Geometry: final body of the model. Coordinates: model frame, mm. Face numbers are marked on the shaded views. A direction names the side the tool comes from. Coordinates: 2 decimals unless noted, no trailing zeros. Loops run counter-clockwise (first coordinate to the right, second up) from the corner with the lowest first, then second, coordinate; pieces in that order, holes last. Notation, with made-up numbers: (12.5, 23) - (68.5, 23) arc R19 ccw to (68.5, 35) - close; hole circle Ø6 at (29.25, -0.5). An arc over 180 degrees is marked (long way). Put each result on its own line as item: value. Start each with the question number.
1) Reachability of the marked faces 1, 2 and 3 from +Z, -Z, +X, -X, +Y, -Y: full face, straight path, thin tool, end or side. Return the list, or none.
2) Contact query for flat-ended pins moving along their axis: pin 1 Ø3 at (y, z) = (9, -25.5) entering from -X; pin 2 Ø10 at (y, z) = (34.5, -19) entering from -X; pin 3 Ø6 at (y, z) = (32, -29) entering from +X; pin 4 Ø3.5 at (x, z) = (61.5, -20) entering from +Y. Output: stop coordinate, or through.
3) Material intervals for line 1 along X through (y, z) = (1, -20); line 2 along X through (y, z) = (39.75, -20); line 3 along Z through (x, y) = (50, 3), sorted ascending. Write a range as from..to.
4) Section D-D on y = 43.5. Output: boundary loops of the cut face in (x, z).
5) Draft query along Y for the marked faces 4, 5, 6 and 7. Return one class per face: +Y half, -Y half, draft (parallel to the pull), parting line (faces both ways), or undercut.
6) Section B-B on x = 35. Output: boundary loops of the cut face in (y, z).
7) Section C-C on y = 29. Output: boundary loops of the cut face in (x, z), and give its area (3 significant figures).
8) Section A-A on z = -20. Output: boundary loops of the cut face in (x, y), and give its area (3 significant figures).
```python
from build123d import *

# Parameters (mm, degrees)
BOSS_EXTRUDE1_DEPTH = 7
SKETCH4_R           = 1.55
CUT_EXTRUDE1_DEPTH  = 89.684835231
SKETCH5_W           = 70
SKETCH5_H           = 8
BOSS_EXTRUDE2_DEPTH = 40
SKETCH6_W           = 20
SKETCH6_H           = 20
CUT_EXTRUDE2_DEPTH  = 101.124921973
BOSS_EXTRUDE4_DEPTH = 46
SKETCH9_R           = 2.6
CUT_EXTRUDE3_DEPTH  = 101.124921973
SKETCH10_W          = 70
SKETCH10_H          = 7
BOSS_EXTRUDE5_DEPTH = 7


with BuildPart() as part:
    # Sketch1 → Boss-Extrude1 (new body)
    with BuildSketch(Plane(origin=(0, 0, 0), x_dir=(1, 0, 0), z_dir=(0, 1, 0))):
        Polygon((0, 54), (0, 0), (15, 0), (15, 41), (55, 41), (55, 0), (70, 0), (70, 54), align=None)
    extrude(amount=BOSS_EXTRUDE1_DEPTH)

    # Sketch4 → Cut-Extrude1 (cut, through all)
    with BuildSketch(Plane(origin=(0, 7, 0), x_dir=(1, 0, 0), z_dir=(0, 1, 0))):
        with Locations(Location((8.5, 20, 0), (0, 0, 270))):
            Circle(SKETCH4_R)
        with Locations(Location((61.5, 20, 0), (0, 0, 270))):
            Circle(SKETCH4_R)
    extrude(amount=-CUT_EXTRUDE1_DEPTH, mode=Mode.SUBTRACT)

    # Sketch5 → Boss-Extrude2 (add)
    with BuildSketch(Plane(origin=(0, 7, 0), x_dir=(1, 0, 0), z_dir=(0, 1, 0))):
        with Locations((35, 50)):
            Rectangle(SKETCH5_W, SKETCH5_H)
    extrude(amount=BOSS_EXTRUDE2_DEPTH)

    # Sketch6 → Cut-Extrude2 (cut, through all)
    with BuildSketch(Plane(origin=(0, 0, -54), x_dir=(-1, 0, 0), z_dir=(0, 0, -1))):
        with Locations((-35, 27)):
            Rectangle(SKETCH6_W, SKETCH6_H)
    extrude(amount=-CUT_EXTRUDE2_DEPTH, mode=Mode.SUBTRACT)

    # Sketch8 → Boss-Extrude4 (add)
    with BuildSketch(Plane.XY.offset(-46)):
        Polygon((18, 47), (52, 47), (52, 27), (45, 27), (45, 37), (25, 37), (25, 27), (18, 27), align=None)
    extrude(amount=BOSS_EXTRUDE4_DEPTH)

    # Sketch9 → Cut-Extrude3 (cut, through all)
    with BuildSketch(Plane(origin=(0, 47, 0), x_dir=(1, 0, 0), z_dir=(0, 1, 0))):
        with Locations(Location((35, 20, 0), (0, 0, 270))):
            Circle(SKETCH9_R)
    extrude(amount=-CUT_EXTRUDE3_DEPTH, mode=Mode.SUBTRACT)

    # Sketch10 → Boss-Extrude5 (add)
    with BuildSketch(Plane.XY):
        with Locations((35, 3.5)):
            Rectangle(SKETCH10_W, SKETCH10_H)
    extrude(amount=BOSS_EXTRUDE5_DEPTH)


solid = part.part
```
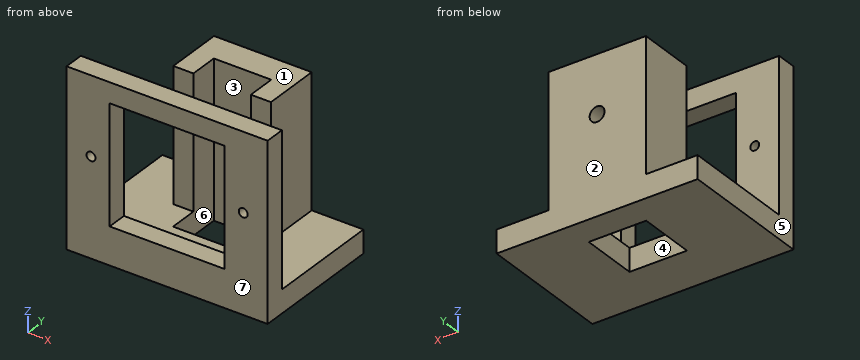
Answer block:
1. face 1: +Z, +X, -X, +Y
1. face 2: +Z, -Z, +X, -X, +Y
1. face 3: +Z, -Z
2. pin 1: passes through
2. pin 2: stops at x = 18
2. pin 3: stops at x = 52
2. pin 4: stops at y = 7
3. line 1: x = 0..6.95, 10.05..15, 55..59.95, 63.05..70
3. line 2: x = 18..32.4, 37.6..52
3. line 3: z = -54..-41, 0..7
4. outline: (0, -54) - (70, -54) - (70, -46) - (52, -46) - (52, 0) - (18, 0) - (18, -46) - (0, -46) - close; hole circle Ø5.2 at (35, -20)
5. face 4: undercut
5. face 5: draft
5. face 6: undercut
5. face 7: -Y half
6. outline: (0, -54) - (17, -54) - (17, -46) - (7, -46) - (7, -41) - (0, -41) - close; (0, 0) - (7, 0) - (7, 7) - (0, 7) - close; (37, -54) - (47, -54) - (47, -22.6) - (37, -22.6) - close; (37, -17.4) - (47, -17.4) - (47, 0) - (37, 0) - close
7. outline: (0, -54) - (25, -54) - (25, 0) - (18, 0) - (18, -46) - (0, -46) - close; (45, -54) - (70, -54) - (70, -46) - (52, -46) - (52, 0) - (45, 0) - close
7. area: 1,040 mm²
8. outline: (0, 0) - (6.95, 0) - (6.95, 7) - (0, 7) - close; (10.05, 0) - (15, 0) - (15, 7) - (10.05, 7) - close; (18, 27) - (25, 27) - (25, 37) - (32.4, 37) - (32.4, 47) - (18, 47) - close; (37.6, 37) - (45, 37) - (45, 27) - (52, 27) - (52, 47) - (37.6, 47) - close; (55, 0) - (59.95, 0) - (59.95, 7) - (55, 7) - close; (63.05, 0) - (70, 0) - (70, 7) - (63.05, 7) - close
8. area: 595 mm²
